```python
from build123d import *

# Parameters (mm, degrees)
F0_W     = 23.8125
F0_H     = 7.9375
F0_R     = 2.54
F1_DEPTH = 7.9375
F3_DEPTH = 7.9375
F4_R     = 3.96874


# Not quite as in the source:
# - a fillet or chamfer is up to 0.001 mm smaller than in the source, because OpenCascade refuses the exact size


with BuildPart() as f1:
    # F0 (on Top) → F1 (new body)
    with BuildSketch(Plane.XY):
        Rectangle(F0_W, F0_H)
        Circle(F0_R, mode=Mode.SUBTRACT)
    extrude(amount=F1_DEPTH)

    # F2 (on face) → F3 (cut, through all)
    with BuildSketch(Plane.XZ.offset(3.96875)):
        with BuildLine():
            ThreePointArc((-5.3975, 3.96875), (-7.9375, 6.50875), (-10.4775, 3.96875))
            Line((-10.4775, 3.96875), (-7.9375, 3.96875))
            Line((-7.9375, 3.96875), (-5.3975, 3.96875))
        make_face()
        with BuildLine():
            ThreePointArc((10.4775, 3.96875), (7.9375, 6.50875), (5.3975, 3.96875))
            Line((5.3975, 3.96875), (7.9375, 3.96875))
            Line((7.9375, 3.96875), (10.4775, 3.96875))
        make_face()
        with BuildLine():
            Line((7.9375, 3.96875), (5.3975, 3.96875))
            ThreePointArc((5.3975, 3.96875), (7.9375, 1.42875), (10.4775, 3.96875))
            Line((10.4775, 3.96875), (7.9375, 3.96875))
        make_face()
        with BuildLine():
            Line((-7.9375, 3.96875), (-10.4775, 3.96875))
            ThreePointArc((-10.4775, 3.96875), (-7.9375, 1.42875), (-5.3975, 3.96875))
            Line((-5.3975, 3.96875), (-7.9375, 3.96875))
        make_face()
    extrude(amount=-F3_DEPTH, mode=Mode.SUBTRACT)

    # F4 (radius 3.96875 in the source; OpenCascade refuses exactly that, so slightly less here)
    f4_edges = [f1.edges().sort_by_distance(p)[0] for p in [
        (11.90625, 0, 7.9375),
        (11.90625, 0, 0),
        (-11.90625, 0, 7.9375),
        (-11.90625, 0, 0),
    ]]
    fillet(f4_edges, radius=F4_R)


solid = f1.part
```
Verification items for the finished model (mm, model axes). Give positions to 0.01 mm unless a question says otherwise; leave off trailing zeros. Write each loop counter-clockwise with the first axis right and the second up, starting at its lowest first coordinate (ties: lowest second). Pieces come first, ordered by that corner, then holes. Notation, with made-up numbers: (28.25, 53) - (57.25, 53) arc R18 ccw to (57.25, 83) - close; hole circle Ø2 at (87, 5.5). An arc over 180 degrees is marked (long way). Put each result on its own line as item: value.
Q1. Section check B-B on z = 3.75. Record the cut outline in (x, y).
Result:
outline: (-11.9, -3.97) - (-10.47, -3.97) - (-10.47, 3.97) - (-11.9, 3.97) - close; (-5.41, -3.97) - (5.41, -3.97) - (5.41, 3.97) - (-5.41, 3.97) - close; (10.47, -3.97) - (11.9, -3.97) - (11.9, 3.97) - (10.47, 3.97) - close; hole circle Ø5.08 at (0, 0)
Q2. Scan lines: probe 1 along X at (y, z) = (3.25, 5); probe 2 along X at (y, z) = (-0.5, 5); probe 3 along X at (y, z) = (1.5, 5). Record each from-to range of solid material in increasing order. Write a range as from..to.
Result:
probe 1: -11.77..-10.26, -5.62..5.62, 10.26..11.77
probe 2: -11.77..-10.26, -5.62..-2.49, 2.49..5.62, 10.26..11.77
probe 3: -11.77..-10.26, -5.62..-2.05, 2.05..5.62, 10.26..11.77
Q3. Depth check by flat-ended pin: P1, Ø1.5, axis at y = 0.5, z = 2.5, coming from the -X side; P2, Ø3, axis at x = -9, y = 1, coming from the -Z side. Enter the tip coordinate at first touch or a pass-through.
Result:
P1: x = -11.84
P2: z = 0
Q4. Section check D-D on x = 0. Record the cut outline in (y, z).
Result:
outline: (-3.97, 0) - (-2.54, 0) - (-2.54, 7.94) - (-3.97, 7.94) - close; (2.54, 0) - (3.97, 0) - (3.97, 7.94) - (2.54, 7.94) - close
Q5. Section check A-A on y = 0. Count the separate pieces of the cut face and the enclosed holes in it, and give its area (3 significant figures).
Result:
separate pieces: 2
enclosed holes: 2
area: 94.6 mm2
Q6. Mould release check, pull along X, two halves, no side actions. Record for faces 1 (the face through (-10.775, 0.056, 6.744)), 2 (the face through (-10.36, -0.06, 3.21)), 3 (the face through (-0.33, 2.52, 3.91)), 4 (the face through (0, -3.969, 4)): released by +X, released by -X, zero draft, split by the parting line, or undercut.
Result:
face 1: released by -X
face 2: undercut
face 3: undercut
face 4: zero draft
